Can you work these out from the model? Positions are in its coordinate system, mm. Face numbers are marked on the shaded views. Coordinates: 2 decimals unless noted, no trailing zeros. Order: outer loops, then holes, each group sorted by start corner. A loop starts at its lowest first (then second) coordinate and runs counter-clockwise, first axis right, second up. Notation, with made-up numbers: M 67,-8.75 L 116,-8.75 A27 cw 116,17.25 Z; hole C 81,-1.75 d4. An arc over 180 degrees is marked long. Answer as CSV lines item,"result". Start each with the question number.
1. If we mould it in two halves opening along X, with no side actions, what happens to the marked faces 1, 2 and 3? For each: released by +X, released by -X, zero draft, split by the parting line, or undercut.
2. If we section it at C-C (y = 8): List the corners of the cut face in (x, z) for me (1 decimal), plus the area to 3 significant figures.
3. Will these pins go through, and if not, where does the flat tip stop? pin 1 (2 mm diameter, centred on x = -13, y = 46.5, fed in from -Z); pin 2 (2 mm diameter, centred on x = -23.01, z = 0, fed in from +Y); pin 3 (8 mm diameter, centred on x = 16, y = 25.5, fed in from +Z); pin 4 (3.5 mm diameter, centred on x = 23.01, z = 0, fed in from -Y) (3 decimals).
4. If we section it at B-B (z = 0): Give the number of separate pieces and of enclosed holes in the cut face, plus the area to 3 significant figures.
5. I need wall thicknesses on line 1 along X through (y, z) = (53.25, 0); line 2 along Z through (x, y) = (-1, 41.5); line 3 along X through (y, z) = (7.75, 0). Which ranges of each line are inside material? Lowest first, please. Write a range as from..to.
6. If we section it at D-D (x = -20.5): List the corners of the cut face in (y, z) for me (3 decimals), plus the area to 3 significant figures.
```python
from build123d import *

# Parameters (mm, degrees)
SKETCH1_R           = 36.5125
SKETCH1_R_2         = 33.3375
BOSS_EXTRUDE1_DEPTH = 51.435
BOSS_EXTRUDE5_START = 6.096
SKETCH6_R           = 36.5125
SKETCH6_R_2         = 33.3375
BOSS_EXTRUDE5_DEPTH = 6.096
SKETCH12_R          = 33.3375
SKETCH12_R_2        = 25.4
BOSS_EXTRUDE8_DEPTH = 28.321
SKETCH2_R           = 36.5125
SKETCH2_R_2         = 19.05
BOSS_EXTRUDE2_DEPTH = 6.35
SKETCH4_R           = 26.9494
CUT_EXTRUDE1_DEPTH  = 1.7272
SKETCH5_R           = 1.1303
CUT_EXTRUDE5_DEPTH  = 83.140778384


with BuildPart() as part:
    # Sketch1 → Boss-Extrude1 (new body)
    with BuildSketch(Plane(origin=(0, 0, 0), x_dir=(1, 0, 0), z_dir=(0, 1, 0))):
        with Locations(Location((0, 0, 0), (0, 0, 270))):
            Circle(SKETCH1_R)
        with Locations(Location((0, 0, 0), (0, 0, 270))):
            Circle(SKETCH1_R_2, mode=Mode.SUBTRACT)
    extrude(amount=BOSS_EXTRUDE1_DEPTH)

    # Sketch6 → Boss-Extrude5 (add)
    with BuildSketch(Plane.XZ.offset(BOSS_EXTRUDE5_START)):
        with Locations(Location((0, 0, 0), (0, 0, 270))):
            Circle(SKETCH6_R)
        with Locations(Location((0, 0, 0), (0, 0, 270))):
            Circle(SKETCH6_R_2, mode=Mode.SUBTRACT)
    extrude(amount=-BOSS_EXTRUDE5_DEPTH)

    # Sketch12 → Boss-Extrude8 (add)
    with BuildSketch(Plane.XZ.offset(-23.114)):
        with Locations(Location((0, 0, 0), (0, 0, 270))):
            Circle(SKETCH12_R)
        with Locations(Location((0, 0, 0), (0, 0, 270))):
            Circle(SKETCH12_R_2, mode=Mode.SUBTRACT)
    extrude(amount=-BOSS_EXTRUDE8_DEPTH)

    # Sketch2 → Boss-Extrude2 (add)
    with BuildSketch(Plane(origin=(0, 51.435, 0), x_dir=(1, 0, 0), z_dir=(0, 1, 0))):
        with Locations(Location((0, 0, 0), (0, 0, 90))):
            Circle(SKETCH2_R)
        with Locations(Location((0, 0, 0), (0, 0, 270))):
            Circle(SKETCH2_R_2, mode=Mode.SUBTRACT)
    extrude(amount=BOSS_EXTRUDE2_DEPTH)

    # Sketch4 → Cut-Extrude1 (cut)
    with BuildSketch(Plane.XZ.offset(-26.67)):
        with Locations(Location((0, 0, 0), (0, 0, 270))):
            Circle(SKETCH4_R)
    extrude(amount=CUT_EXTRUDE1_DEPTH, mode=Mode.SUBTRACT)

    # Sketch5 → Cut-Extrude5 (cut, through all)
    with BuildSketch(Plane(origin=(0, 57.785, 0), x_dir=(1, 0, 0), z_dir=(0, 1, 0))):
        with Locations(Location((-23.0124, 0, 0), (0, 0, 270))):
            Circle(SKETCH5_R)
        with Locations(Location((23.0124, 0, 0), (0, 0, 270))):
            Circle(SKETCH5_R)
    extrude(amount=-CUT_EXTRUDE5_DEPTH, mode=Mode.SUBTRACT)


solid = part.part
```
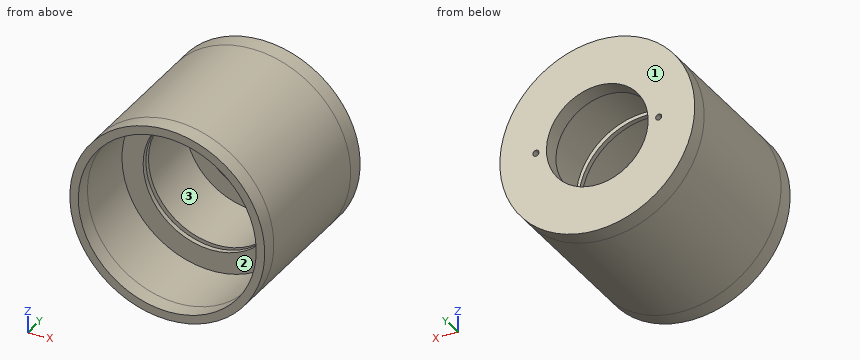
Solved:
1,face 1,"zero draft"
1,face 2,"undercut"
1,face 3,"undercut"
2,outline,"C 0,0 d73; hole C 0,0 d66.7"
2,area,"697 mm²"
3,pin 1,"z = -34.48"
3,pin 2,"through"
3,pin 3,"z = 34.48"
3,pin 4,"y = 51.435"
4,separate pieces,"4"
4,enclosed holes,"0"
4,area,"1,000 mm²"
5,line 1,"-36.51..-24.14, -21.88..-19.05, 19.05..21.88, 24.14..36.51"
5,line 2,"-36.5..-25.38, 25.38..36.5"
5,line 3,"-36.51..-33.34, 33.34..36.51"
6,outline,"M -6.096,-30.214 L 57.785,-30.214 L 57.785,30.214 L -6.096,30.214 L -6.096,26.29 L 23.114,26.29 L 23.114,14.997 L 24.943,14.997 L 24.943,17.493 L 26.67,17.493 L 26.67,14.997 L 51.435,14.997 L 51.435,-14.997 L 26.67,-14.997 L 26.67,-17.493 L 24.943,-17.493 L 24.943,-14.997 L 23.114,-14.997 L 23.114,-26.29 L -6.096,-26.29 Z"
6,area,"1,470 mm²"
